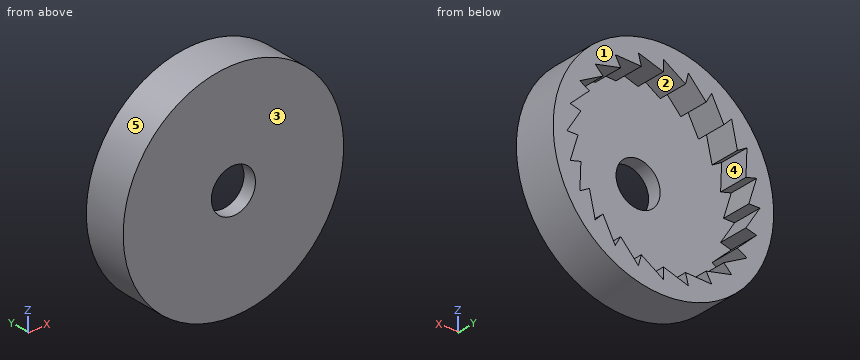
from build123d import *

# Parameters (mm, degrees)
SKETCH1_R           = 20
SKETCH1_R_2         = 17.5
BOSS_EXTRUDE2_DEPTH = 8
SHELL2_T            = -2.5
BOSS_EXTRUDE3_DEPTH = 5.5
SKETCH4_R           = 4
CUT_EXTRUDE1_DEPTH  = 12


with BuildPart() as part:
    # Sketch1 → Boss-Extrude2 (new body)
    # profile 1 of 2: a face of its own
    with BuildSketch(Plane(origin=(0, 0, 0), x_dir=(1, 0, 0), z_dir=(0, 1, 0))):
        with Locations(Location((0, 0, 0), (0, 0, 270))):
            Circle(SKETCH1_R)
        Circle(SKETCH1_R_2, mode=Mode.SUBTRACT)
    # profile 2 of 2: a face of its own
    with BuildSketch(Plane(origin=(0, 0, 0), x_dir=(1, 0, 0), z_dir=(0, 1, 0))):
        Circle(SKETCH1_R_2)
    extrude(amount=BOSS_EXTRUDE2_DEPTH)

    # Shell2
    shell2_openings = [part.faces().sort_by_distance(p)[0] for p in [
        (0, 8, 0),
    ]]
    offset(amount=SHELL2_T, openings=shell2_openings, kind=Kind.INTERSECTION)

    # Sketch3 → Boss-Extrude3 (add)
    with BuildSketch(Plane(origin=(0, 2.5, 0), x_dir=(1, 0, 0), z_dir=(0, 1, 0))):
        with BuildLine():
            Line((-14.971850307, -4.011695199), (-16.90370196, -4.529333289))
            ThreePointArc((-16.90370196, -4.529333289), (-16.167891819, -6.696960066), (-15.155444566, -8.75))
            Line((-15.155444566, -8.75), (-14.971850307, -4.011695199))
        make_face()
        with BuildLine():
            Line((-15.5, 0), (-17.5, 0))
            ThreePointArc((-17.5, 0), (-17.350285074, -2.284208364), (-16.90370196, -4.529333289))
            Line((-16.90370196, -4.529333289), (-15.5, 0))
        make_face()
        with BuildLine():
            Line((-14.971850307, 4.011695199), (-16.90370196, 4.529333289))
            ThreePointArc((-16.90370196, 4.529333289), (-17.350285074, 2.284208364), (-17.5, 0))
            Line((-17.5, 0), (-14.971850307, 4.011695199))
        make_face()
        with BuildLine():
            ThreePointArc((0, 17.5), (-2.284208364, 17.350285074), (-4.529333289, 16.90370196))
            Line((-4.529333289, 16.90370196), (0, 15.5))
            Line((0, 15.5), (0, 17.5))
        make_face()
        with BuildLine():
            ThreePointArc((4.529333289, 16.90370196), (2.284208364, 17.350285074), (0, 17.5))
            Line((0, 17.5), (4.011695199, 14.971850307))
            Line((4.011695199, 14.971850307), (4.529333289, 16.90370196))
        make_face()
        with BuildLine():
            ThreePointArc((8.75, 15.155444566), (6.696960066, 16.167891819), (4.529333289, 16.90370196))
            Line((4.529333289, 16.90370196), (7.75, 13.423393759))
            Line((7.75, 13.423393759), (8.75, 15.155444566))
        make_face()
        with BuildLine():
            ThreePointArc((12.374368671, 12.374368671), (10.653325008, 13.883683455), (8.75, 15.155444566))
            Line((8.75, 15.155444566), (10.960155108, 10.960155108))
            Line((10.960155108, 10.960155108), (12.374368671, 12.374368671))
        make_face()
        with BuildLine():
            ThreePointArc((15.155444566, 8.75), (13.883683455, 10.653325008), (12.374368671, 12.374368671))
            Line((12.374368671, 12.374368671), (13.423393759, 7.75))
            Line((13.423393759, 7.75), (15.155444566, 8.75))
        make_face()
        with BuildLine():
            ThreePointArc((16.90370196, 4.529333289), (16.167891819, 6.696960066), (15.155444566, 8.75))
            Line((15.155444566, 8.75), (14.971850307, 4.011695199))
            Line((14.971850307, 4.011695199), (16.90370196, 4.529333289))
        make_face()
        with BuildLine():
            ThreePointArc((17.5, 0), (17.350285074, 2.284208364), (16.90370196, 4.529333289))
            Line((16.90370196, 4.529333289), (15.5, 0))
            Line((15.5, 0), (17.5, 0))
        make_face()
        with BuildLine():
            ThreePointArc((16.90370196, -4.529333289), (17.350285074, -2.284208364), (17.5, 0))
            Line((17.5, 0), (14.971850307, -4.011695199))
            Line((14.971850307, -4.011695199), (16.90370196, -4.529333289))
        make_face()
        with BuildLine():
            ThreePointArc((15.155444566, -8.75), (16.167891819, -6.696960066), (16.90370196, -4.529333289))
            Line((16.90370196, -4.529333289), (13.423393759, -7.75))
            Line((13.423393759, -7.75), (15.155444566, -8.75))
        make_face()
        with BuildLine():
            ThreePointArc((12.374368671, -12.374368671), (13.883683455, -10.653325008), (15.155444566, -8.75))
            Line((15.155444566, -8.75), (10.960155108, -10.960155108))
            Line((10.960155108, -10.960155108), (12.374368671, -12.374368671))
        make_face()
        with BuildLine():
            ThreePointArc((8.75, -15.155444566), (10.653325008, -13.883683455), (12.374368671, -12.374368671))
            Line((12.374368671, -12.374368671), (7.75, -13.423393759))
            Line((7.75, -13.423393759), (8.75, -15.155444566))
        make_face()
        with BuildLine():
            ThreePointArc((4.529333289, -16.90370196), (6.696960066, -16.167891819), (8.75, -15.155444566))
            Line((8.75, -15.155444566), (4.011695199, -14.971850307))
            Line((4.011695199, -14.971850307), (4.529333289, -16.90370196))
        make_face()
        with BuildLine():
            Line((0, -15.5), (0, -17.5))
            ThreePointArc((0, -17.5), (2.284208364, -17.350285074), (4.529333289, -16.90370196))
            Line((4.529333289, -16.90370196), (0, -15.5))
        make_face()
        with BuildLine():
            Line((-4.011695199, -14.971850307), (-4.529333289, -16.90370196))
            ThreePointArc((-4.529333289, -16.90370196), (-2.284208364, -17.350285074), (0, -17.5))
            Line((0, -17.5), (-4.011695199, -14.971850307))
        make_face()
        with BuildLine():
            Line((-7.75, -13.423393759), (-8.75, -15.155444566))
            ThreePointArc((-8.75, -15.155444566), (-6.696960066, -16.167891819), (-4.529333289, -16.90370196))
            Line((-4.529333289, -16.90370196), (-7.75, -13.423393759))
        make_face()
        with BuildLine():
            Line((-10.960155108, -10.960155108), (-12.374368671, -12.374368671))
            ThreePointArc((-12.374368671, -12.374368671), (-10.653325008, -13.883683455), (-8.75, -15.155444566))
            Line((-8.75, -15.155444566), (-10.960155108, -10.960155108))
        make_face()
        with BuildLine():
            Line((-13.423393759, -7.75), (-15.155444566, -8.75))
            ThreePointArc((-15.155444566, -8.75), (-13.883683455, -10.653325008), (-12.374368671, -12.374368671))
            Line((-12.374368671, -12.374368671), (-13.423393759, -7.75))
        make_face()
        with BuildLine():
            Line((-13.423393759, 7.75), (-15.155444566, 8.75))
            ThreePointArc((-15.155444566, 8.75), (-16.167891819, 6.696960066), (-16.90370196, 4.529333289))
            Line((-16.90370196, 4.529333289), (-13.423393759, 7.75))
        make_face()
        with BuildLine():
            Line((-10.960155108, 10.960155108), (-12.374368671, 12.374368671))
            ThreePointArc((-12.374368671, 12.374368671), (-13.883683455, 10.653325008), (-15.155444566, 8.75))
            Line((-15.155444566, 8.75), (-10.960155108, 10.960155108))
        make_face()
        with BuildLine():
            Line((-7.75, 13.423393759), (-8.75, 15.155444566))
            ThreePointArc((-8.75, 15.155444566), (-10.653325008, 13.883683455), (-12.374368671, 12.374368671))
            Line((-12.374368671, 12.374368671), (-7.75, 13.423393759))
        make_face()
        with BuildLine():
            Line((-4.011695199, 14.971850307), (-4.529333289, 16.90370196))
            ThreePointArc((-4.529333289, 16.90370196), (-6.696960066, 16.167891819), (-8.75, 15.155444566))
            Line((-8.75, 15.155444566), (-4.011695199, 14.971850307))
        make_face()
    extrude(amount=BOSS_EXTRUDE3_DEPTH)

    # Sketch4 → Cut-Extrude1 (cut)
    with BuildSketch(Plane(origin=(0, 2.5, 0), x_dir=(1, 0, 0), z_dir=(0, 1, 0))):
        with Locations(Location((0, 0, 0), (0, 0, 270))):
            Circle(SKETCH4_R)
    extrude(amount=-CUT_EXTRUDE1_DEPTH, mode=Mode.SUBTRACT)


solid = part.part
CAD build for the part. Positions are in the model's coordinates, mm. Face numbers are marked on the shaded views. A direction names the side the tool comes from. Give positions to 0.01 mm unless a question says otherwise; leave off trailing zeros. Order: outer loops, then holes, each group sorted by start corner. A loop starts at its lowest first (then second) coordinate and runs counter-clockwise, first axis right, second up. Notation, with made-up numbers: (71, 18.25) - (110, 18.25) arc R20 ccw to (110, 24.25) - close; hole circle Ø10 at (70.25, -15.5). An arc over 180 degrees is marked (long way). Write each question's results on one line, items separated by ' | '.
1. Saw through at B-B on z = 3. List the corners of the cut face in (x, y).
Calculated:
outline: (-19.77, 0) - (-2.65, 0) - (-2.65, 2.5) - (-16.43, 2.5) - (-16.43, 8) - (-19.77, 8) - close; (2.65, 0) - (19.77, 0) - (19.77, 8) - (15.61, 8) - (15.61, 2.5) - (2.65, 2.5) - close
2. Probe L1, parallel to X at y = 1.95, z = 0; L2, parallel to Y at x = 4, z = 13; L3, parallel to X at y = 6, z = 1.5. List the from-to ranges inside material, lowest first. Write a range as from..to.
Calculated:
L1: x = -20..-4, 4..20 | L2: y = 0..2.5 | L3: x = -19.94..-15.96, 16.55..19.94
3. Saw through at C-C on y = 2. List the corners of the cut face in (x, z).
Calculated:
outline: circle Ø40 at (0, 0); hole circle Ø8 at (0, 0)
4. 3-axis set-ups, long thin cutter, end or side, ignore diameter. For the marked faces 1 and 2: which of +Z, -Z, +X, -X, +Y, -Y reach the whole face in a straight line?
Calculated:
face 1: +Z, -Z, +X, -X, +Y | face 2: +Y
5. Saw through at D-D on z = -7. List the corners of the cut face in (x, y) (3 decimals), and give its area (3 significant figures).
Calculated:
outline: (-18.735, 0) - (18.735, 0) - (18.735, 8) - (15.088, 8) - (15.088, 2.5) - (-14.234, 2.5) - (-14.234, 8) - (-18.735, 8) - close | area: 138 mm2
6. Pin check, flat tips, straight feed: pin 1 (17.5 mm diameter, centred on x = 8.5, z = -4.5, fed in from +Y); pin 2 (6 mm diameter, centred on x = -2, z = -12.5, fed in from +Y); pin 3 (4 mm diameter, centred on x = 11, y = 1.5, fed in from -Z); pin 4 (1.6 mm diameter, centred on y = 4, z = -17, fed in from +X). Stop position of each tip, or through.
Calculated:
pin 1: stops at y = 8 | pin 2: stops at y = 2.5 | pin 3: stops at z = -17.86 | pin 4: stops at x = 11.73
7. Saw through at A-A on x = -0.5. List the corners of the cut face in (y, z), and give its area (3 significant figures).
Calculated:
outline: (0, -19.99) - (8, -19.99) - (8, -15.65) - (2.5, -15.65) - (2.5, -3.97) - (0, -3.97) - close; (0, 3.97) - (2.5, 3.97) - (2.5, 17.18) - (8, 17.18) - (8, 19.99) - (0, 19.99) - close | area: 119 mm2
8. Pull direction Z, two halves, no side cores. Call the marked faces 3, 4 and 5: released by +Z, released by -Z, zero draft, split by the parting line, or undercut.
Calculated:
face 3: zero draft | face 4: undercut | face 5: split by the parting line
